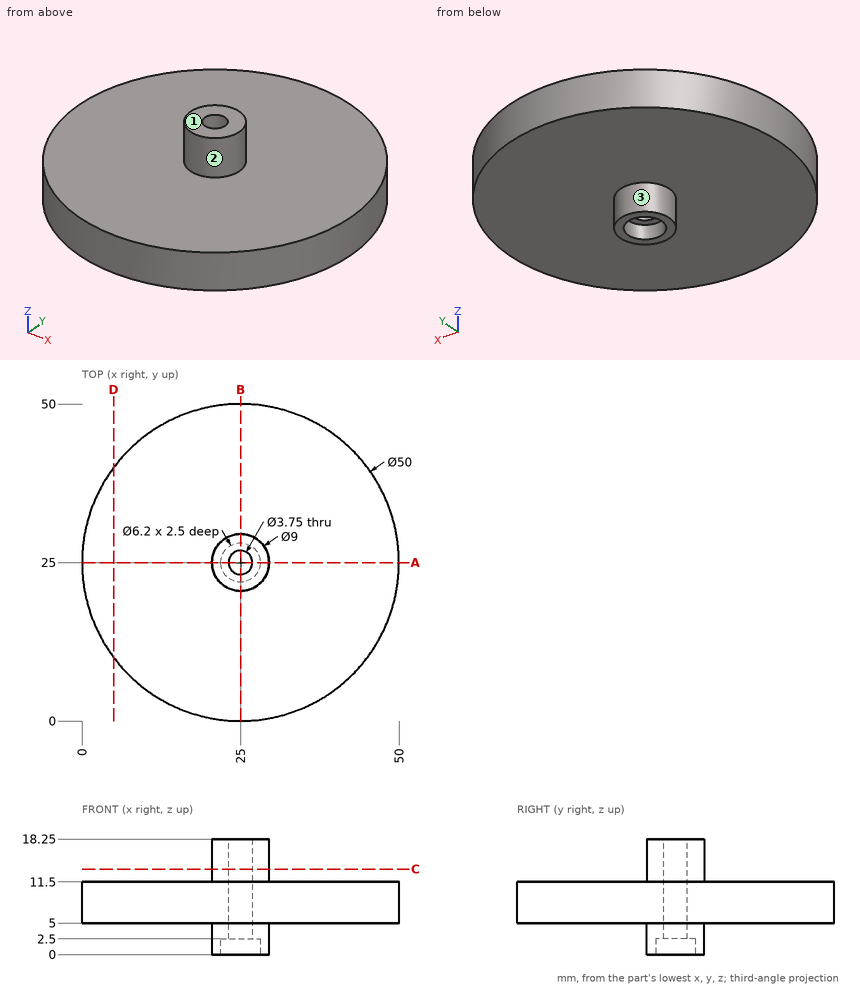
Geometry check sheet. Reference: drawing and pictorial views, mm from the part's lowest x, y, z. A direction names the side the tool comes from. Round coordinates to 2 decimals unless told otherwise and drop trailing zeros. Write each loop counter-clockwise with the first axis right and the second up, starting at its lowest first coordinate (ties: lowest second). Pieces come first, ordered by that corner, then holes.
(1) Material ranges on line 1 (Y direction, x = 25, z = 13) (3 decimals); line 2 (Y direction, x = 25, z = 1.85); line 3 (Z direction, x = 9, y = 21), recorded low to high.
Returned:
line 1: y = 20.5 to 23.125, 26.875 to 29.5
line 2: y = 20.5 to 21.9, 28.1 to 29.5
line 3: z = 5 to 11.5
(2) Section check C-C (z = 13.5). Enter the section's corners in (x, y) (3 decimals), plus the area to 3 significant figures.
Returned:
outline: circle Ø9 at (25, 25); hole circle Ø3.75 at (25, 25)
area: 52.6 mm2
(3) Section check A-A (y = 25). Enter the section's corners in (x, z) (3 decimals), plus the area to 3 significant figures.
Returned:
outline: (0, 5) - (20.5, 5) - (20.5, 0) - (21.9, 0) - (21.9, 2.5) - (23.125, 2.5) - (23.125, 18.25) - (20.5, 18.25) - (20.5, 11.5) - (0, 11.5) - close; (26.875, 2.5) - (28.1, 2.5) - (28.1, 0) - (29.5, 0) - (29.5, 5) - (50, 5) - (50, 11.5) - (29.5, 11.5) - (29.5, 18.25) - (26.875, 18.25) - close
area: 356 mm2
(4) Depth check by flat-ended pin: pin 1 Ø1.5 at (x, z) = (41.5, 11) entering from -Y; pin 2 Ø3 at (x, y) = (25, 25) entering from +Z; pin 3 Ø3 at (x, z) = (13.5, 5) entering from +Y; pin 4 Ø5 at (y, z) = (37, 6) entering from +X. Enter the tip coordinate at first touch or a pass-through.
Returned:
pin 1: stops at y = 5.59
pin 2: passes through
pin 3: stops at y = 47.91
pin 4: stops at x = 48.12
(5) Access from +Z, -Z, +X, -X, +Y, -Y to the whole of each face (thin tool, end or side, straight path). Record for the marked faces 1, 2 and 3.
Returned:
face 1: +Z, +X, -X, +Y, -Y
face 2: +Z
face 3: -Z
(6) Section check D-D (x = 5). Enter the section's corners in (y, z), plus the area to 3 significant figures.
Returned:
outline: (10, 5) - (40, 5) - (40, 11.5) - (10, 11.5) - close
area: 195 mm2
